Part model, mm, in its own coordinate system. A direction names the side the tool comes from. Give positions to 0.01 mm unless a question says otherwise; leave off trailing zeros. Write each loop counter-clockwise with the first axis right and the second up, starting at its lowest first coordinate (ties: lowest second). Pieces come first, ordered by that corner, then holes. Notation, with made-up numbers: M 70,39 L 88,39 A25 ccw 88,52 Z; hole C 44,51 d8. An arc over 180 degrees is marked long. Use a Markdown table: item, result.
Autodesk Inventor part; units mm, degrees
ref_plane "YZ Plane" through (0, 0, 0) normal (1, 0, 0) x (0, 1, 0)
ref_plane "XZ Plane" through (0, 0, 0) normal (0, 1, 0) x (-1, 0, 0)
ref_plane "XY Plane" through (0, 0, 0) normal (0, 0, 1) x (1, 0, 0)
sketch "Náčrt1" plane through (0, 0, 0) normal (0, 1, 0) x (-1, 0, 0)
  line L0 (49.75, -49.75) -> (-49.75, -49.75)
  line L1 (-49.75, -49.75) -> (-49.75, 49.75)
  line L2 (-49.75, 49.75) -> (49.75, 49.75)
  line L3 (49.75, 49.75) -> (49.75, -49.75)
  line L4 (49.75, -49.75) -> (0, 0) construction
  line L5 (0, 0) -> (-49.75, -49.75) construction
  line L6 (0, 0) -> (-49.75, 49.75) construction
  line L7 (50.75, -50.75) -> (-50.75, -50.75)
  line L8 (-50.75, -50.75) -> (-50.75, 50.75)
  line L9 (-50.75, 50.75) -> (50.75, 50.75)
  line L10 (50.75, 50.75) -> (50.75, -50.75)
  dimension "d0" = 99.5
  dimension "d3" = 1
extrude "Vysunutí1" add sketch "Náčrt1" along normal blind 1 contours L0 L1 L2 L3
extrude "Vysunutí2" add sketch "Náčrt1" along normal blind 5
properties part number "box"
1. Tool access for faces 4 (the flat face through (1, 0, 1)), 5 (the flat face through (1, 3, 49.75)): list every direction of +Z, -Z, +X, -X, +Y, -Y with a clear straight run to the whole face (end or side of a thin tool).
Findings below:
| item | result |
|---|---|
| face 4 | +Z, -Z, +X, -X, -Y |
| face 5 | +Y |
2. Cut at A-A, the plane y = 3.8. Give the cut face in (x, z), then the cut area to 3 significant figures.
Findings below:
| item | result |
|---|---|
| outline | M -50.75,-50.75 L 50.75,-50.75 L 50.75,50.75 L -50.75,50.75 Z; hole M -49.75,-49.75 L 49.75,-49.75 L 49.75,49.75 L -49.75,49.75 Z |
| area | 402 mm2 |
3. Cut at B-B, the plane x = 15. Give the cut face in (y, z), then the cut area to 4 significant figures.
Findings below:
| item | result |
|---|---|
| outline | M 0,-50.75 L 5,-50.75 L 5,-49.75 L 1,-49.75 L 1,49.75 L 5,49.75 L 5,50.75 L 0,50.75 Z |
| area | 109.5 mm2 |
4. Drop flat-ended pins along their axis: P1, Ø3, axis at x = 6.5, z = -25, coming from the -Y side; P2, Ø1, axis at x = -8, z = -11.5, coming from the +Y side. Give the stop position or say it passes through.
Findings below:
| item | result |
|---|---|
| P1 | y = 0 |
| P2 | y = 1 |
5. Two-plate mould, pull along X, no slides. Class faces 1 (the flat face through (-1, 2, -50.75)), 2 (the flat face through (1, 1, 1)), 3 (the flat face through (-50.75, 2, 1)): released by +X, released by -X, zero draft, split by the parting line, or undercut.
Findings below:
| item | result |
|---|---|
| face 1 | zero draft |
| face 2 | undercut |
| face 3 | released by -X |
6. Drill centre lines: L1, parallel to Z at x = -6.5, y = 4.45; L2, parallel to Y at x = 41, z = 32.5. Where is each one in solid material? Low to high.
Findings below:
| item | result |
|---|---|
| L1 | -50.75 to -49.75, 49.75 to 50.75 |
| L2 | 0 to 1 |
7. Cut at C-C, the plane z = -38. Give the cut face in (x, y).
Findings below:
| item | result |
|---|---|
| outline | M -50.75,0 L 50.75,0 L 50.75,5 L 49.75,5 L 49.75,1 L -49.75,1 L -49.75,5 L -50.75,5 Z |
